The drawing under review shows one solid part. Ordinate dimensions are in mm from its lowest x, y, z. A direction names the side the tool comes from. Give positions to 0.01 mm unless a question says otherwise; leave off trailing zeros. Write each loop counter-clockwise with the first axis right and the second up, starting at its lowest first coordinate (ties: lowest second). Pieces come first, ordered by that corner, then holes.
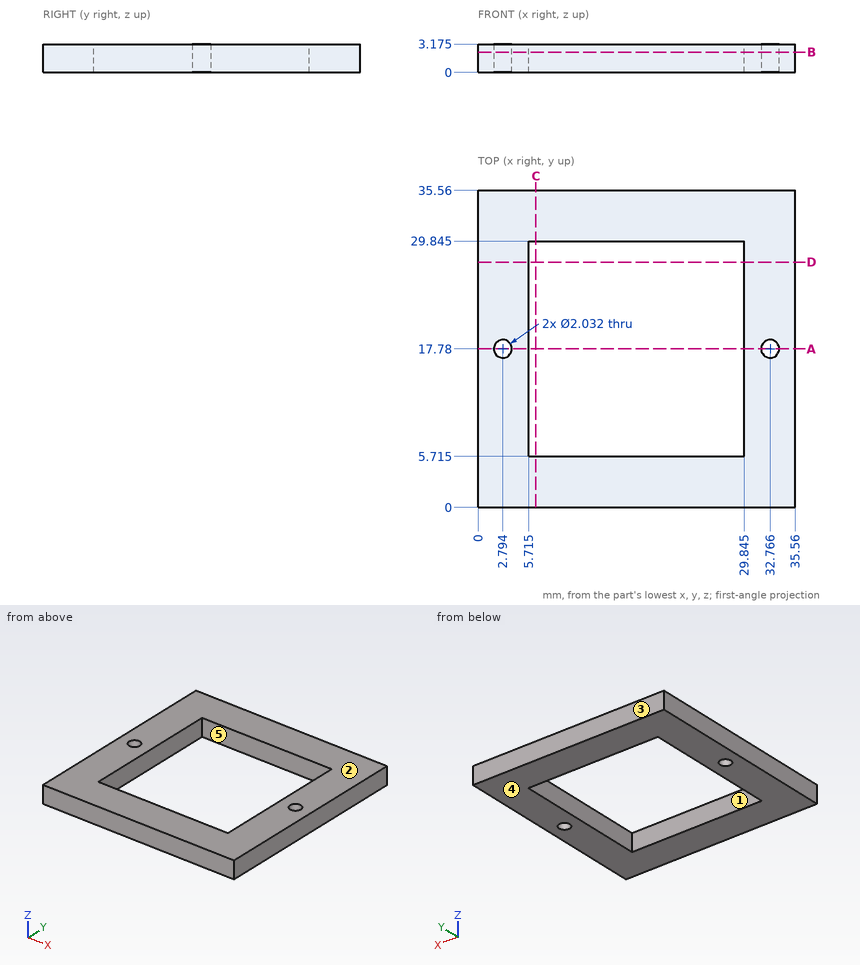
1) The part is to be moulded in two halves that separate along Y. For the marked faces 3, 4 and 5, say which applies: +Y half, -Y half, draft (parallel to the pull), parting line (faces both ways), or undercut.
2) Insertion check: pin 1 (1.6 mm diameter, centred on y = 20, z = 2, fed in from -X). The pin has a flat end and moves straight along its axis. Give the tip position at first contact, or say it passes through.
3) To check wall thickness, follow probe 1 along X at (y, z) = (25, 0.3) (3 decimals); probe 2 along X at (y, z) = (18, 2.7) (3 decimals). State the ranges of each line that lie inside material, in increasing order.
4) Consider section A-A, the plane y = 17.78. Give the boundary of the cut face in (x, z) (3 decimals).
5) Consider section C-C, the plane x = 6.5. Give the boundary of the cut face in (y, z) (3 decimals), then the cut area to 3 significant figures.
6) Tool access review of the marked faces 1 and 2: name each direction out of +Z, -Z, +X, -X, +Y, -Y from which nothing blocks a thin tool from reaching the whole face with its end or side.
7) Consider section B-B, the plane z = 2.25. Give the boundary of the cut face in (x, y) (3 decimals), then the cut area to 3 significant figures.
Answer block:
1. face 3: +Y half
1. face 4: draft
1. face 5: undercut
2. pin 1: stops at x = 0
3. probe 1: x = 0 to 5.715, 29.845 to 35.56
3. probe 2: x = 0 to 1.802, 3.786 to 5.715, 29.845 to 31.774, 33.758 to 35.56
4. outline: (0, 0) - (1.778, 0) - (1.778, 3.175) - (0, 3.175) - close; (3.81, 0) - (5.715, 0) - (5.715, 3.175) - (3.81, 3.175) - close; (29.845, 0) - (31.75, 0) - (31.75, 3.175) - (29.845, 3.175) - close; (33.782, 0) - (35.56, 0) - (35.56, 3.175) - (33.782, 3.175) - close
5. outline: (0, 0) - (5.715, 0) - (5.715, 3.175) - (0, 3.175) - close; (29.845, 0) - (35.56, 0) - (35.56, 3.175) - (29.845, 3.175) - close
5. area: 36.3 mm2
6. face 1: +Z, -Z
6. face 2: +Z, +X, -X, +Y, -Y
7. outline: (0, 0) - (35.56, 0) - (35.56, 35.56) - (0, 35.56) - close; hole circle Ø2.032 at (2.794, 17.78); hole (5.715, 5.715) - (29.845, 5.715) - (29.845, 29.845) - (5.715, 29.845) - close; hole circle Ø2.032 at (32.766, 17.78)
7. area: 676 mm2
